Drawing for the job (mm, zero at the part's lowest x, y, z). A direction names the side the tool comes from. Give positions to 0.01 mm unless a question says otherwise; leave off trailing zeros. Write each loop counter-clockwise with the first axis right and the second up, starting at its lowest first coordinate (ties: lowest second). Pieces come first, ordered by that corner, then holes. Notation, with made-up numbers: (11.25, -5.5) - (50.25, -5.5) arc R28 cw to (50.25, 25.5) - close; hole circle Ø9 at (77.5, 37). An arc over 180 degrees is marked (long way). Answer as a JSON object with one key per item and string values. Group by question number.
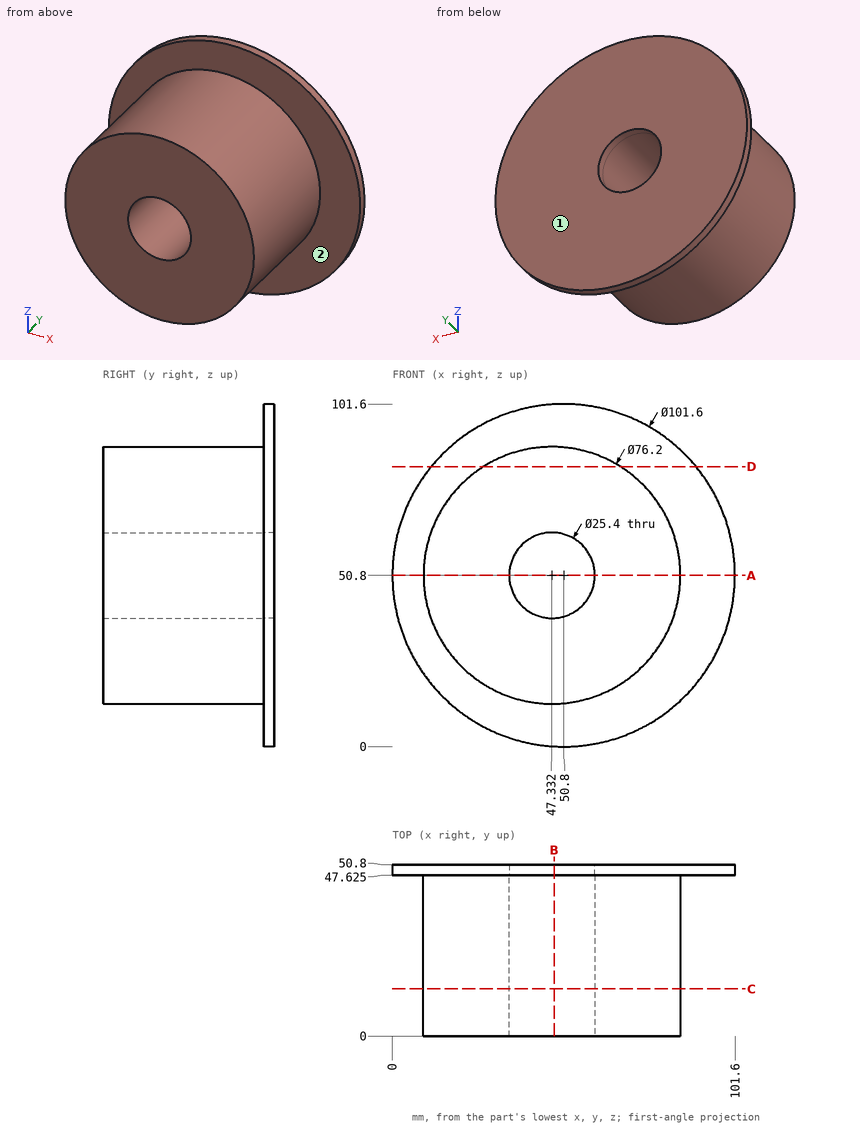
1) Band-saw the part on A-A (z = 50.8). List the corners of the cut face in (x, y) (1 decimal), plus the area to 3 significant figures.
2) Which spindle directions (+Z, -Z, +X, -X, +Y, -Y) get a long thin tool onto all of the face, cutting with end or side? Do the marked faces 1 and 2. Say none if no direction does.
3) Probe line 1 (X direction, y = 35, z = 50); line 2 (X direction, y = 49, z = 50); line 3 (Y direction, x = 81, z = 73) (3 decimals). List the from-to ranges inside material, lowest first.
4) Band-saw the part on D-D (z = 83). List the corners of the cut face in (x, y) (1 decimal), plus the area to 3 significant figures.
5) Band-saw the part on C-C (y = 14). List the corners of the cut face in (x, z), plus the area to 3 significant figures.
6) Band-saw the part on B-B (x = 48). List the corners of the cut face in (y, z) (1 decimal), plus the area to 3 significant figures.
7) Drop flat-ended pins along their axis: P1, Ø1, axis at x = 68, y = 18, coming from the -Z side; P2, Ø12, axis at x = 41.5, y = 36, coming from the +Z side; P3, Ø8, axis at y = 31, z = 16.5, coming from the -X side. Give the stop position or say it passes through.
Verdict:
{
 "1": {"outline": "(0, 47.6) - (9.2, 47.6) - (9.2, 0) - (34.6, 0) - (34.6, 50.8) - (0, 50.8) - close; (60, 0) - (85.4, 0) - (85.4, 47.6) - (101.6, 47.6) - (101.6, 50.8) - (60, 50.8) - close", "area": "2,660 mm2"},
 "2": {"face 1": "+Z, -Z, +X, -X, +Y", "face 2": "-Y"},
 "3": {"line 1": "9.24 to 34.66, 60.01 to 85.42", "line 2": "0.01 to 34.66, 60.01 to 101.59", "line 3": "47.625 to 50.8"},
 "4": {"outline": "(11.5, 47.6) - (27, 47.6) - (27, 0) - (67.7, 0) - (67.7, 47.6) - (90.1, 47.6) - (90.1, 50.8) - (11.5, 50.8) - close", "area": "2,190 mm2"},
 "5": {"outline": "circle Ø76.2 at (47.33, 50.8); hole circle Ø25.4 at (47.33, 50.8)", "area": "4,050 mm2"},
 "6": {"outline": "(0, 12.7) - (47.6, 12.7) - (47.6, 0.1) - (50.8, 0.1) - (50.8, 38.1) - (0, 38.1) - close; (0, 63.5) - (50.8, 63.5) - (50.8, 101.5) - (47.6, 101.5) - (47.6, 88.9) - (0, 88.9) - close", "area": "2,660 mm2"},
 "7": {"P1": "z = 18.48", "P2": "z = 88.9", "P3": "x = 24.23"}
}
